from build123d import *

# Parameters (mm, degrees)
BOSS_EXTRUDE1_DEPTH = 3
CUT_EXTRUDE1_DEPTH  = 3
SKETCH10_R          = 1.5
CUT_EXTRUDE2_DEPTH  = 4
SKETCH11_R          = 1.5
CUT_EXTRUDE3_DEPTH  = 4
SKETCH12_R          = 1.5
CUT_EXTRUDE4_DEPTH  = 10
SKETCH13_R          = 1.5
CUT_EXTRUDE5_DEPTH  = 10
SKETCH15_R          = 1.5
CUT_EXTRUDE6_DEPTH  = 10
SKETCH16_R          = 4
SKETCH16_R_2        = 1.5
BOSS_EXTRUDE3_DEPTH = 3


with BuildPart() as part:
    # Sketch1 → Boss-Extrude1 (new body)
    with BuildSketch(Plane.XY):
        with BuildLine():
            Line((-254.850919962, 60.230742329), (36.781104638, 60.230742329))
            Line((36.781104638, 60.230742329), (36.781104638, -7.509642512))
            ThreePointArc((36.781104638, -7.509642512), (7.803285657, -54.719658484), (50.224189815, -90.342214419))
            Line((50.224189815, -90.342214419), (82.677328038, -89.923825571))
            Line((82.677328038, -89.923825571), (82.677328038, -97.923825571))
            Line((82.677328038, -97.923825571), (-254.850919962, -97.923825571))
            Line((-254.850919962, -97.923825571), (-254.850919962, 60.230742329))
        make_face()
    extrude(amount=BOSS_EXTRUDE1_DEPTH)

    # Sketch3 → Cut-Extrude1 (cut)
    with BuildSketch(Plane.XY.offset(3)):
        Polygon((67.728416495, -97.923825571), (67.728416495, -90.116548316), (82.677328038, -89.923825571), (82.677328038, -97.923825571), align=None)
    extrude(amount=-CUT_EXTRUDE1_DEPTH, mode=Mode.SUBTRACT)

    # Sketch10 → Cut-Extrude2 (cut)
    with BuildSketch(Plane.XY.offset(3)):
        with Locations((-2.442671962, -11.923825571)):
            Circle(SKETCH10_R)
        with Locations((-2.442671962, -63.923825571)):
            Circle(SKETCH10_R)
    extrude(amount=-CUT_EXTRUDE2_DEPTH, mode=Mode.SUBTRACT)

    # Sketch11 → Cut-Extrude3 (cut)
    with BuildSketch(Plane.XY.offset(3)):
        with Locations((-70.942671962, 35.507538029)):
            Circle(SKETCH11_R)
        with Locations((-70.942671962, -70.492461971)):
            Circle(SKETCH11_R)
    extrude(amount=-CUT_EXTRUDE3_DEPTH, mode=Mode.SUBTRACT)

    # Sketch12 → Cut-Extrude4 (cut)
    with BuildSketch(Plane.XY.offset(3)):
        with Locations((-6.43991594, 56.230742329)):
            Circle(SKETCH12_R)
        with Locations((6.56008406, 56.230742329)):
            Circle(SKETCH12_R)
        with Locations((6.56008406, 7.430742329)):
            Circle(SKETCH12_R)
        with Locations((-6.43991594, 7.430742329)):
            Circle(SKETCH12_R)
    extrude(amount=-CUT_EXTRUDE4_DEPTH, mode=Mode.SUBTRACT)

    # Sketch13 → Cut-Extrude5 (cut)
    with BuildSketch(Plane.XY.offset(3)):
        with Locations((-145.230919962, 35.230742329)):
            Circle(SKETCH13_R)
        with Locations((-145.230919962, -72.923825571)):
            Circle(SKETCH13_R)
    extrude(amount=-CUT_EXTRUDE5_DEPTH, mode=Mode.SUBTRACT)

    # Sketch15 → Cut-Extrude6 (cut)
    with BuildSketch(Plane.XY.offset(3)):
        with Locations((-252.350919962, -72.919257671)):
            Circle(SKETCH15_R)
        with Locations((-252.350919962, 35.226174429)):
            Circle(SKETCH15_R)
    extrude(amount=-CUT_EXTRUDE6_DEPTH, mode=Mode.SUBTRACT)

    # Sketch16 → Boss-Extrude3 (add)
    # profile 1 of 2: a face of its own
    with BuildSketch(Plane.XY.offset(3)):
        with Locations((-252.350919962, -72.919257671)):
            Circle(SKETCH16_R)
        with Locations((-252.350919962, -72.919257671)):
            Circle(SKETCH16_R_2, mode=Mode.SUBTRACT)
    # profile 2 of 2: a face of its own
    with BuildSketch(Plane.XY.offset(3)):
        with Locations((-252.350919962, 35.226174429)):
            Circle(SKETCH16_R)
        with Locations((-252.350919962, 35.226174429)):
            Circle(SKETCH16_R_2, mode=Mode.SUBTRACT)
    extrude(amount=-BOSS_EXTRUDE3_DEPTH)


solid = part.part
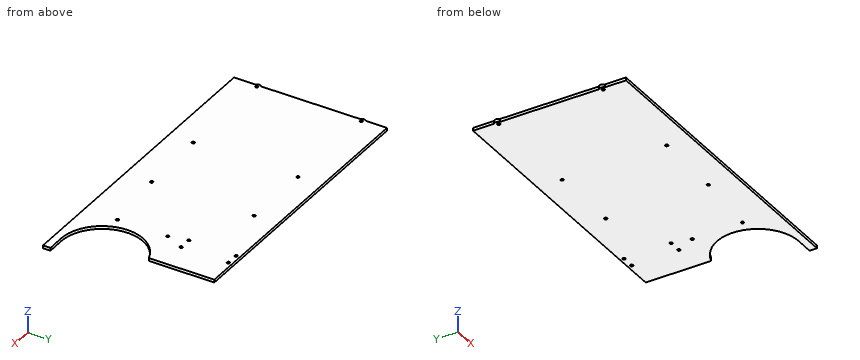
The listing builds one solid part. Answer for the finished solid, in the listing's coordinates (mm). Coordinates: 2 decimals unless noted, no trailing zeros. Write each loop counter-clockwise with the first axis right and the second up, starting at its lowest first coordinate (ties: lowest second). Pieces come first, ordered by that corner, then holes. Notation, with made-up numbers: (-9, 39.25) - (4, 39.25) arc R20 cw to (4, 51.25) - close; hole circle Ø5 at (72, -16.75). An arc over 180 degrees is marked (long way). Answer as CSV lines item,"result".
1. Given P1, Ø1.5, axis at y = -34, z = 2, coming from the -X side; P2, Ø1.8, axis at x = -252.35, y = -72.92, coming from the -Z side, each flat-ended and moving along its own axis, determine where each tip first touches the part or whether it passes through.
Computed values:
P1,"stops at x = -254.85"
P2,"passes through"
2. Find section C-C (y = -21). Give the vertices of the cut face in (x, z), plus the area to 3 significant figures.
Computed values:
outline,"(-254.85, 0) - (16.89, 0) - (16.89, 3) - (-254.85, 3) - close"
area,"815 mm²"
3. Straight lines are drawn through the part: line 1 (X direction, y = 35.5, z = 1.55); line 2 (X direction, y = 7, z = 2.7); line 3 (X direction, y = 42, z = 1.3). For each, find the intervals that lie inside material, in ascending order. Write a range as [from, to].
Computed values:
line 1,"x = [-256.34, -253.83], [-250.88, -146.71], [-143.76, -72.44], [-69.44, 36.78]"
line 2,"x = [-254.85, -7.88], [-5, 5.12], [8, 36.78]"
line 3,"x = [-254.85, 36.78]"
4. Find section A-A (z = 1.75). Give the number of separate pieces and of enclosed holes in the cut face, plus the area to 3 significant figures.
Computed values:
separate pieces,"1"
enclosed holes,"12"
area,"44,500 mm²"
5. Find section B-B (y = 29). Give the vertices of the cut face in (x, z).
Computed values:
outline,"(-254.85, 0) - (36.78, 0) - (36.78, 3) - (-254.85, 3) - close"
